from build123d import *

# Parameters (mm, degrees)
SKETCH1_W           = 15
SKETCH1_H           = 15
BOSS_EXTRUDE1_DEPTH = 8
BOSS_EXTRUDE2_DEPTH = 18
BOSS_EXTRUDE3_START = -2
BOSS_EXTRUDE3_DEPTH = 2


with BuildPart() as part:
    # Sketch1 → Boss-Extrude1 (new body)
    with BuildSketch(Plane(origin=(0, 0, 0), x_dir=(1, 0, 0), z_dir=(0, 1, 0))):
        with BuildLine():
            Line((-77, 40), (77, 40))
            ThreePointArc((77, 40), (79.121320344, 39.121320344), (80, 37))
            Line((80, 37), (80, -37))
            ThreePointArc((80, -37), (79.121320344, -39.121320344), (77, -40))
            Line((77, -40), (-77, -40))
            ThreePointArc((-77, -40), (-79.121320344, -39.121320344), (-80, -37))
            Line((-80, -37), (-80, 37))
            ThreePointArc((-80, 37), (-79.121320344, 39.121320344), (-77, 40))
        make_face()
        with Locations((-46, 24.5)):
            Rectangle(SKETCH1_W, SKETCH1_H, mode=Mode.SUBTRACT)
        with Locations((-64.5, 24.5)):
            Rectangle(SKETCH1_W, SKETCH1_H, mode=Mode.SUBTRACT)
        with Locations((-27.5, 24.5)):
            Rectangle(SKETCH1_W, SKETCH1_H, mode=Mode.SUBTRACT)
        with Locations((-9, 24.5)):
            Rectangle(SKETCH1_W, SKETCH1_H, mode=Mode.SUBTRACT)
        with Locations((9.5, 24.5)):
            Rectangle(SKETCH1_W, SKETCH1_H, mode=Mode.SUBTRACT)
        with Locations((28, 24.5)):
            Rectangle(SKETCH1_W, SKETCH1_H, mode=Mode.SUBTRACT)
        with Locations((46.5, 24.5)):
            Rectangle(SKETCH1_W, SKETCH1_H, mode=Mode.SUBTRACT)
        with Locations((65, 24.5)):
            Rectangle(SKETCH1_W, SKETCH1_H, mode=Mode.SUBTRACT)
        with Locations((-46, 0.5)):
            Rectangle(SKETCH1_W, SKETCH1_H, mode=Mode.SUBTRACT)
        with Locations((-27.5, 0.5)):
            Rectangle(SKETCH1_W, SKETCH1_H, mode=Mode.SUBTRACT)
        with Locations((-9, 0.5)):
            Rectangle(SKETCH1_W, SKETCH1_H, mode=Mode.SUBTRACT)
        with Locations((9.5, 0.5)):
            Rectangle(SKETCH1_W, SKETCH1_H, mode=Mode.SUBTRACT)
        with Locations((28, 0.5)):
            Rectangle(SKETCH1_W, SKETCH1_H, mode=Mode.SUBTRACT)
        with Locations((46.5, 0.5)):
            Rectangle(SKETCH1_W, SKETCH1_H, mode=Mode.SUBTRACT)
        with Locations((65, 0.5)):
            Rectangle(SKETCH1_W, SKETCH1_H, mode=Mode.SUBTRACT)
        with Locations((-46, -23.5)):
            Rectangle(SKETCH1_W, SKETCH1_H, mode=Mode.SUBTRACT)
        with Locations((-27.5, -23.5)):
            Rectangle(SKETCH1_W, SKETCH1_H, mode=Mode.SUBTRACT)
        with Locations((-9, -23.5)):
            Rectangle(SKETCH1_W, SKETCH1_H, mode=Mode.SUBTRACT)
        with Locations((9.5, -23.5)):
            Rectangle(SKETCH1_W, SKETCH1_H, mode=Mode.SUBTRACT)
        with Locations((28, -23.5)):
            Rectangle(SKETCH1_W, SKETCH1_H, mode=Mode.SUBTRACT)
        with Locations((46.5, -23.5)):
            Rectangle(SKETCH1_W, SKETCH1_H, mode=Mode.SUBTRACT)
        with Locations((65, -23.5)):
            Rectangle(SKETCH1_W, SKETCH1_H, mode=Mode.SUBTRACT)
        with Locations((-64.5, 0.5)):
            Rectangle(SKETCH1_W, SKETCH1_H, mode=Mode.SUBTRACT)
        with Locations((-64.5, -23.5)):
            Rectangle(SKETCH1_W, SKETCH1_H, mode=Mode.SUBTRACT)
    extrude(amount=BOSS_EXTRUDE1_DEPTH)

    # Sketch1_3 → Boss-Extrude2 (add)
    with BuildSketch(Plane(origin=(0, 0, 0), x_dir=(1, 0, 0), z_dir=(0, 1, 0))):
        with BuildLine():
            Line((-77, 40), (77, 40))
            ThreePointArc((77, 40), (79.121320344, 39.121320344), (80, 37))
            Line((80, 37), (80, -37))
            ThreePointArc((80, -37), (79.121320344, -39.121320344), (77, -40))
            Line((77, -40), (-77, -40))
            ThreePointArc((-77, -40), (-79.121320344, -39.121320344), (-80, -37))
            Line((-80, -37), (-80, 37))
            ThreePointArc((-80, 37), (-79.121320344, 39.121320344), (-77, 40))
        make_face()
        with BuildLine():
            Line((-72, 35), (72, 35))
            ThreePointArc((72, 35), (74.121320344, 34.121320344), (75, 32))
            Line((75, 32), (75, -32))
            ThreePointArc((75, -32), (74.121320344, -34.121320344), (72, -35))
            Line((72, -35), (-72, -35))
            ThreePointArc((-72, -35), (-74.121320344, -34.121320344), (-75, -32))
            Line((-75, -32), (-75, 32))
            ThreePointArc((-75, 32), (-74.121320344, 34.121320344), (-72, 35))
        make_face(mode=Mode.SUBTRACT)
    extrude(amount=BOSS_EXTRUDE2_DEPTH)

    # Sketch1_4 → Boss-Extrude3 (add)
    with BuildSketch(Plane(origin=(0, 0, 0), x_dir=(1, 0, 0), z_dir=(0, 1, 0)).offset(BOSS_EXTRUDE3_START)):
        with BuildLine():
            Line((-77, 40), (77, 40))
            ThreePointArc((77, 40), (79.121320344, 39.121320344), (80, 37))
            Line((80, 37), (80, -37))
            ThreePointArc((80, -37), (79.121320344, -39.121320344), (77, -40))
            Line((77, -40), (-77, -40))
            ThreePointArc((-77, -40), (-79.121320344, -39.121320344), (-80, -37))
            Line((-80, -37), (-80, 37))
            ThreePointArc((-80, 37), (-79.121320344, 39.121320344), (-77, 40))
        make_face()
    extrude(amount=BOSS_EXTRUDE3_DEPTH)


solid = part.part
Model file for the job. Use its own axes, mm. A direction names the side the tool comes from. Give positions to 0.01 mm unless a question says otherwise; leave off trailing zeros. Order: outer loops, then holes, each group sorted by start corner. A loop starts at its lowest first (then second) coordinate and runs counter-clockwise, first axis right, second up. Notation, with made-up numbers: (62.25, 89.5) - (75.25, 89.5) arc R19 ccw to (75.25, 124.5) - close; hole circle Ø2 at (-9.5, 68). An arc over 180 degrees is marked (long way). Return JSON: item names as keys, results as strings.
1) Flat gauge pins, fed straight in: P1, Ø4.5, axis at x = -30.5, z = -23, coming from the +Y side; P2, Ø12, axis at x = -66.5, z = 1.5, coming from the +Y side. Where does each tip first touch, or does it go through?
Geometry says:
{"P1": "y = 0", "P2": "y = 8"}
2) Cut at B-B, the plane z = 11.5. Give the cut face in (x, y), plus the area to 3 significant figures.
Geometry says:
{"outline": "(-80, -2) - (80, -2) - (80, 18) - (75, 18) - (75, 8) - (-75, 8) - (-75, 18) - (-80, 18) - close", "area": "1,700 mm²"}
3) Probe line 1 (Z direction, x = 15, y = 2.25); line 2 (Z direction, x = 65, y = 12.25); line 3 (X direction, y = 15.5, z = -1). List the from-to ranges inside material, lowest first. Write a range as from..to.
Geometry says:
{"line 1": "-40..-32, -17..-8, 7..16, 31..40", "line 2": "-40..-35, 35..40", "line 3": "-80..-75, 75..80"}
4) 3-axis set-ups, long thin cutter, end or side, ignore diameter. For faces 1 (the flat face through (1, -2, -1)), 2 (the flat face through (65, 0, -25)): which of +Z, -Z, +X, -X, +Y, -Y reach the whole face in a straight line?
Geometry says:
{"face 1": "+Z, -Z, +X, -X, -Y", "face 2": "+Y"}
5) Cut at A-A, the plane y = 10. Give the cut face in (x, z), plus the area to 3 significant figures.
Geometry says:
{"outline": "(-80, -37) arc R3 ccw to (-77, -40) - (77, -40) arc R3 ccw to (80, -37) - (80, 37) arc R3 ccw to (77, 40) - (-77, 40) arc R3 ccw to (-80, 37) - close; hole (-75, -32) arc R3 ccw to (-72, -35) - (72, -35) arc R3 ccw to (75, -32) - (75, 32) arc R3 ccw to (72, 35) - (-72, 35) arc R3 ccw to (-75, 32) - close", "area": "2,300 mm²"}
6) Pull direction X, two halves, no side cores. Call faces 3 (the flat face through (1, 8, 40)), 4 (the flat face through (80, 8, -1)), 5 (the flat face through (-72, 4, 0)): pulls with the +X half, pulls with the -X half, needs draft (parallel to the pull), parting line crosses it, or undercut.
Geometry says:
{"face 3": "needs draft", "face 4": "pulls with the +X half", "face 5": "undercut"}
7) Cut at C-C, the plane x = 37.5. Give the cut face in (y, z).
Geometry says:
{"outline": "(-2, -40) - (18, -40) - (18, -35) - (8, -35) - (8, 35) - (18, 35) - (18, 40) - (-2, 40) - close"}
8) Cut at D-D, the plane x = 15.5. Give the cut face in (y, z), plus the area to 3 significant figures.
Geometry says:
{"outline": "(-2, -40) - (18, -40) - (18, -35) - (8, -35) - (8, -32) - (0, -32) - (0, -17) - (8, -17) - (8, -8) - (0, -8) - (0, 7) - (8, 7) - (8, 16) - (0, 16) - (0, 31) - (8, 31) - (8, 35) - (18, 35) - (18, 40) - (-2, 40) - close", "area": "540 mm²"}
